Verification items for the finished model (mm, model axes). A direction names the side the tool comes from. Coordinates: 2 decimals unless noted, no trailing zeros. Loops run counter-clockwise (first coordinate to the right, second up) from the corner with the lowest first, then second, coordinate; pieces in that order, holes last. Notation, with made-up numbers: (88, 25) -> (122, 25) arc R32 cw to (122, 62) -> close; hole circle Ø3 at (78.5, -39). An arc over 180 degrees is marked (long way). Answer as a JSON object with one key per item and string values. Group by question number.
Q1. Cross-section at A-A on z = 5.5. Give the number of separate pieces and of enclosed holes in the cut face, and give its area (3 significant figures).
Q2. Release check for a two-part mould opening along X. For faces 6 (the cylindrical face through (16, 30, 5)), 7 (the cylindrical face through (59, 2, 5)), 8 (the cylindrical face through (62, 14, 5)) record: released by +X, released by -X, zero draft, split by the parting line, or undercut.
Q3. Gauge pin test, flat ends, axial feed: pin 1 Ø2 at (y, z) = (24.5, 4.5) entering from -X; pin 2 Ø3 at (x, z) = (209.5, 5.5) entering from -Y; pin 3 Ø5 at (x, z) = (108.5, 7) entering from -Y. Record the tip position at first contact, or that the pin passes through.
Q4. Cross-section at B-B on x = 224. Record the boundary of the cut face in (y, z).
Q5. Scan lines: L1, parallel to Y at x = 7.5, z = 5; L2, parallel to Y at x = 40, z = 3; L3, parallel to X at y = 8.5, z = 3.75. Record each from-to range of solid material in increasing order.
Q6. Cross-section at C-C on x = 108. Record the boundary of the cut face in (y, z).
Q7. Set-up check for faces 1 (the flat face through (185, 53, 5)), 2 (the cylindrical face through (6, 53, 3)), 3 (the flat face through (121, 30, 10)), 4 (the cylindrical face through (184, 13, 5)), 5 (the flat face through (121, 30, 0)): record each of +Z, -Z, +X, -X, +Y, -Y from which the full face is reachable in a straight line by a thin tool's end or side.
```python
from build123d import *

# Parameters (mm, degrees)
BOSS_EXTRUDE1_DEPTH = 10
SKETCH2_R           = 2
SKETCH2_R_2         = 16
CUT_EXTRUDE1_DEPTH  = 11
FILLET1_R           = 5
SKETCH3_R           = 2
CUT_EXTRUDE2_DEPTH  = 11
SKETCH4_W           = 10
SKETCH4_H           = 60
CUT_EXTRUDE3_DEPTH  = 246
SKETCH5_R           = 2
CUT_EXTRUDE4_DEPTH  = 12


with BuildPart() as part:
    # Sketch1 → Boss-Extrude1 (new body)
    with BuildSketch(Plane.XY):
        Polygon((245, 5), (245, 55), (185, 55), (185, 45), (60, 45), (60, 60), (-60, 60), (-60, 45), (-185, 45), (-185, 55), (-245, 55), (-245, 5), (-185, 5), (-185, 15), (-60, 15), (-60, 0), (60, 0), (60, 15), (185, 15), (185, 5), align=None)
    extrude(amount=BOSS_EXTRUDE1_DEPTH)

    # Sketch2 → Cut-Extrude1 (cut, through all)
    with BuildSketch(Plane.XY.offset(10)):
        with Locations((40, 20)):
            Circle(SKETCH2_R)
        with Locations((40, 40)):
            Circle(SKETCH2_R)
        with Locations((-40, 40)):
            Circle(SKETCH2_R)
        with Locations((-40, 20)):
            Circle(SKETCH2_R)
        with Locations((0, 30)):
            Circle(SKETCH2_R_2)
    extrude(amount=-CUT_EXTRUDE1_DEPTH, mode=Mode.SUBTRACT)

    # Fillet1
    fillet1_edges = [part.edges().sort_by_distance(p)[0] for p in [
        (185, 15, 5),
        (60, 15, 5),
        (60, 0, 5),
        (-60, 0, 5),
        (-60, 15, 5),
        (-185, 15, 5),
        (-185, 45, 5),
        (-60, 45, 5),
        (-60, 60, 5),
        (60, 60, 5),
        (60, 45, 5),
        (185, 45, 5),
    ]]
    fillet(fillet1_edges, radius=FILLET1_R)

    # Sketch3 → Cut-Extrude2 (cut, through all)
    with BuildSketch(Plane.XY.offset(10)):
        with Locations((-125, 30)):
            Circle(SKETCH3_R)
        with Locations((125, 30)):
            Circle(SKETCH3_R)
    extrude(amount=-CUT_EXTRUDE2_DEPTH, mode=Mode.SUBTRACT)

    # Sketch4 → Cut-Extrude3 (cut, through all)
    with BuildSketch(Plane(origin=(0, 0, 0), x_dir=(0, 0, -1), z_dir=(1, 0, 0))):
        with Locations((-5, 30)):
            Rectangle(SKETCH4_W, SKETCH4_H)
    extrude(amount=-CUT_EXTRUDE3_DEPTH, mode=Mode.SUBTRACT)

    # Sketch5 → Cut-Extrude4 (cut)
    with BuildSketch(Plane.ZY):
        with Locations((5, 53)):
            Circle(SKETCH5_R)
        with Locations((5, 7)):
            Circle(SKETCH5_R)
    extrude(amount=-CUT_EXTRUDE4_DEPTH, mode=Mode.SUBTRACT)


solid = part.part
```
Computed values:
{
 "1": {"separate pieces": "1", "enclosed holes": "3", "area": "9,830 mm²"},
 "2": {"face 6": "released by -X", "face 7": "released by +X", "face 8": "undercut"},
 "3": {"pin 1": "stops at x = 14.62", "pin 2": "stops at y = 5", "pin 3": "stops at y = 15"},
 "4": {"outline": "(5, 0) -> (55, 0) -> (55, 10) -> (5, 10) -> close"},
 "5": {"L1": "y = 0 to 5, 9 to 15.87, 44.13 to 51, 55 to 60", "L2": "y = 0 to 18, 22 to 38, 42 to 60", "L3": "x = 12 to 60, 185 to 245"},
 "6": {"outline": "(15, 0) -> (45, 0) -> (45, 10) -> (15, 10) -> close"},
 "7": {"face 1": "+Z, -Z, +Y", "face 2": "-X", "face 3": "+Z, +X, -X, +Y, -Y", "face 4": "+Z, -Z, -Y", "face 5": "-Z, +X, -X, +Y, -Y"}
}
